Verification items for the finished model (mm, model axes). A direction names the side the tool comes from. Round coordinates to 2 decimals unless told otherwise and drop trailing zeros. Order: outer loops, then holes, each group sorted by start corner. A loop starts at its lowest first (then second) coordinate and runs counter-clockwise, first axis right, second up. Notation, with made-up numbers: (34, -36.75) -> (38, -36.75) arc R18 ccw to (38, -16.75) -> close; hole circle Ø7 at (0.25, -38.5). An arc over 180 degrees is marked (long way). Return JSON: item names as keys, results as strings. Group by question number.
Item 1: Sectioned sample at B-B on x = 0. Record the cut outline in (y, z), plus the area to 3 significant figures.
Item 2: Scan lines: probe 1 along Y at (x, z) = (0, -4); probe 2 along X at (y, z) = (9, 0); probe 3 along Z at (x, y) = (-3.5, 73). Record each from-to range of solid material in increasing order. Write a range as from..to.
Item 3: Sectioned sample at A-A on y = 197. Record the cut outline in (x, z), plus the area to 3 significant figures.
Item 4: Access from +Z, -Z, +X, -X, +Y, -Y to the whole of each face (thin tool, end or side, straight path). Record for faces 1 (the flat face through (0, 20, 0)), 2 (the flat face through (-1, 126, -20)), 3 (the flat face through (77.5, 126, 0)), 4 (the cylindrical face through (3.252, 182.357, -10.14)).
Item 5: Depth check by flat-ended pin: pin 1 Ø12 at (x, y) = (61.5, 142) entering from -Z; pin 2 Ø12 at (y, z) = (155.5, -5.5) entering from -X; pin 3 Ø3 at (x, y) = (3.5, 116.5) entering from +Z; pin 4 Ø8 at (y, z) = (64, 26) entering from +X. Enter the tip coordinate at first touch or a pass-through.
Item 6: Draft check along X on faces 5 (the flat face through (-1, 217, 0)), 6 (the cylindrical face through (0.66, 9.86, 14.985)), 7 (the flat face through (-77.5, 126, 0)). Enter one of: pulls with the +X half, pulls with the -X half, needs draft (parallel to the pull), parting line crosses it, or undercut.
Item 7: Sectioned sample at C-C on y = 125. Record the cut outline in (x, z).
```python
from build123d import *

# Parameters (mm, degrees)
SKETCH2_R           = 90
BOSS_EXTRUDE1_DEPTH = 37
CHAMFER1_SIZE       = 6
SKETCH3_W           = 155
SKETCH3_H           = 40
BOSS_EXTRUDE2_DEPTH = 180
SKETCH30_R          = 15
CUT_EXTRUDE1_DEPTH  = 20
SKETCH31_R          = 15
CUT_EXTRUDE2_DEPTH  = 20


with BuildPart() as part:
    # Sketch2 → Boss-Extrude1 (new body)
    with BuildSketch(Plane(origin=(0, 0, 0), x_dir=(1, 0, 0), z_dir=(0, 1, 0))):
        with Locations(Location((0, 0, 0), (0, 0, 270))):
            Circle(SKETCH2_R)
    extrude(amount=BOSS_EXTRUDE1_DEPTH)

    # Chamfer1
    chamfer1_edges = [part.edges().sort_by_distance(p)[0] for p in [
        (0, 37, -90),
    ]]
    chamfer(chamfer1_edges, length=CHAMFER1_SIZE)

    # Sketch3 → Boss-Extrude2 (add)
    with BuildSketch(Plane(origin=(0, 37, 0), x_dir=(1, 0, 0), z_dir=(0, 1, 0))):
        Rectangle(SKETCH3_W, SKETCH3_H)
    extrude(amount=BOSS_EXTRUDE2_DEPTH)

    # Sketch30 → Cut-Extrude1 (cut)
    with BuildSketch(Plane.XZ):
        with Locations(Location((0, 0, 0), (0, 0, 270))):
            Circle(SKETCH30_R)
    extrude(amount=-CUT_EXTRUDE1_DEPTH, mode=Mode.SUBTRACT)

    # Sketch31 → Cut-Extrude2 (cut)
    with BuildSketch(Plane(origin=(0, 0, -20), x_dir=(-1, 0, 0), z_dir=(0, 0, -1))):
        with Locations((0, 197)):
            Circle(SKETCH31_R)
    extrude(amount=-CUT_EXTRUDE2_DEPTH, mode=Mode.SUBTRACT)


solid = part.part
```
Recorded:
{
 "1": {"outline": "(0, -90) -> (31, -90) -> (37, -84) -> (37, -20) -> (182, -20) -> (182, 0) -> (212, 0) -> (212, -20) -> (217, -20) -> (217, 20) -> (37, 20) -> (37, 84) -> (31, 90) -> (0, 90) -> (0, 15) -> (20, 15) -> (20, -15) -> (0, -15) -> close", "area": "12,600 mm²"},
 "2": {"probe 1": "20..182, 212..217", "probe 2": "-90..-15, 15..90", "probe 3": "-20..20"},
 "3": {"outline": "(-77.5, -20) -> (-15, -20) -> (-15, 0) -> (15, 0) -> (15, -20) -> (77.5, -20) -> (77.5, 20) -> (-77.5, 20) -> close", "area": "5,600 mm²"},
 "4": {"face 1": "-Y", "face 2": "-Z, +X, -X, +Y", "face 3": "+Z, -Z, +X, +Y", "face 4": "-Z"},
 "5": {"pin 1": "z = -20", "pin 2": "x = -77.5", "pin 3": "z = 20", "pin 4": "through"},
 "6": {"face 5": "needs draft", "face 6": "undercut", "face 7": "pulls with the -X half"},
 "7": {"outline": "(-77.5, -20) -> (77.5, -20) -> (77.5, 20) -> (-77.5, 20) -> close"}
}
